```python
from build123d import *

# Parameters (mm, degrees)
F0_R     = 8.5
F1_DEPTH = 18
F1_TAPER = 8
F2_R     = 4
F3_DEPTH = 6.1
F5_DEPTH = 10.6
F6_R     = 2.2
F7_DEPTH = 9.4


with BuildPart() as f1:
    # F0 (on Top) → F1 (new body)
    with BuildSketch(Plane.XY):
        Circle(F0_R)
    extrude(amount=-F1_DEPTH, taper=F1_TAPER)

    # F2 (on Top) → F3 (join)
    with BuildSketch(Plane.XY):
        Circle(F2_R)
    extrude(amount=F3_DEPTH)

    # F4 (on face) → F5 (join)
    with BuildSketch(Plane.XY.offset(6.1)):
        Polygon((0, -3.3139905451), (2.87, -1.6569952726), (2.87, 1.6569952726), (0, 3.3139905451), (-2.87, 1.6569952726), (-2.87, -1.6569952726), align=None)
    extrude(amount=F5_DEPTH)

    # F6 (on face) → F7 (join)
    with BuildSketch(Plane.XY.offset(16.7)):
        Circle(F6_R)
    extrude(amount=F7_DEPTH)


solid = f1.part
```
CAD build for the part. Positions are in the model's coordinates, mm. A direction names the side the tool comes from. Give positions to 0.01 mm unless a question says otherwise; leave off trailing zeros. Write each loop counter-clockwise with the first axis right and the second up, starting at its lowest first coordinate (ties: lowest second). Pieces come first, ordered by that corner, then holes. Notation, with made-up numbers: M 66,-1 L 84,-1 A14 cw 84,20 Z; hole C 48,-10.5 d4. An arc over 180 degrees is marked long. Return JSON: item names as keys, results as strings. Group by question number.
(1) 3-axis set-ups, long thin cutter, end or side, ignore diameter. For faces 1 (the face through (-0.867, -3.905, 3.007)), 2 (the face through (1.46, 2.47, 11.33)), 3 (the face through (-1.46, -2.47, 11.33)), 4 (the face through (-1.41, 2.5, 11.33)): which of +Z, -Z, +X, -X, +Y, -Y reach the whole face in a straight line?
(2) Band-saw the part on A-A (z = 11). Give the cut face in (x, y).
(3) Band-saw the part on B-B (z = 1). Give the cut face in (x, y), and give its area (3 significant figures).
(4) Flat gauge pins, fed straight in: pin 1 Ø1 at (x, z) = (-5, -7.5) entering from +Y; pin 2 Ø1.5 at (x, z) = (-1, 10) entering from -Y; pin 3 Ø1.5 at (x, z) = (-4, 18.5) entering from -Y; pin 4 Ø2.5 at (y, z) = (0, 11.5) entering from +X. Where does each tip first touch, or does it go through?
(5) Band-saw the part on C-C (z = -13). Give the cut face in (x, y).
(6) Drill centre lines: L1, parallel to Z at x = -4.5, y = 2.75; L2, parallel to X at y = -0.5, z = 14; L3, parallel to Y at x = -3.75, z = -12. Where is each one in solid material? Low to high. Write a range as [from, to].
Entries:
{
 "1": {"face 1": "+Z", "face 2": "+Z, +X, +Y", "face 3": "+Z, -X, -Y", "face 4": "+Z, -X, +Y"},
 "2": {"outline": "M -2.87,-1.66 L 0,-3.31 L 2.87,-1.66 L 2.87,1.66 L 0,3.31 L -2.87,1.66 Z"},
 "3": {"outline": "C 0,0 d8", "area": "50.3 mm^2"},
 "4": {"pin 1": "stops at y = 5.94", "pin 2": "stops at y = -3.17", "pin 3": "passes through", "pin 4": "stops at x = 2.87"},
 "5": {"outline": "C 0,0 d13.35"},
 "6": {"L1": "z = [-18, 0]", "L2": "x = [-2.87, 2.87]", "L3": "y = [-5.69, 5.69]"}
}
